```python
from build123d import *

# Parameters (mm, degrees)
SKETCH1_R               = 16
SKETCH1_R_2             = 2
BOSS_EXTRUDE1_DEPTH     = 5
SKETCH2_R               = 7.5
BOSS_EXTRUDE2_DEPTH     = 18.5
CUT_EXTRUDE1_DEPTH      = 33.622844756
CUT_EXTRUDE1_DEPTH_BACK = 33.622844756
SKETCH3_R               = 4


with BuildPart() as part:
    # Sketch1 → Boss-Extrude1 (new body)
    with BuildSketch(Plane(origin=(0, 0, 0), x_dir=(0, 0, -1), z_dir=(1, 0, 0))):
        Circle(SKETCH1_R)
        with Locations((0, 12)):
            Circle(SKETCH1_R_2, mode=Mode.SUBTRACT)
        with Locations((12, 0)):
            Circle(SKETCH1_R_2, mode=Mode.SUBTRACT)
        with Locations((0, -12)):
            Circle(SKETCH1_R_2, mode=Mode.SUBTRACT)
        with Locations((-12, 0)):
            Circle(SKETCH1_R_2, mode=Mode.SUBTRACT)
    extrude(amount=BOSS_EXTRUDE1_DEPTH)

    # Sketch2 → Boss-Extrude2 (add)
    with BuildSketch(Plane(origin=(5, 0, 0), x_dir=(0, 0, -1), z_dir=(1, 0, 0))):
        Circle(SKETCH2_R)
    extrude(amount=BOSS_EXTRUDE2_DEPTH)

    # Sketch3 → Cut-Extrude1 (cut, two sides: drawn at the far end of the back side and taken through both)
    with BuildSketch(Plane.ZY.offset(-CUT_EXTRUDE1_DEPTH_BACK)):
        Circle(SKETCH3_R)
    extrude(amount=CUT_EXTRUDE1_DEPTH + CUT_EXTRUDE1_DEPTH_BACK, mode=Mode.SUBTRACT)


solid = part.part
```
Input: part model. Units: mm. Frame: model coordinates. A direction names the side the tool comes from. Round coordinates to 2 decimals unless told otherwise and drop trailing zeros. Write each loop counter-clockwise with the first axis right and the second up, starting at its lowest first coordinate (ties: lowest second). Pieces come first, ordered by that corner, then holes. Notation, with made-up numbers: M 14,12 L 42,12 A13 ccw 42,24 Z; hole C 65.25,82.25 d9. An arc over 180 degrees is marked long. Write each question's results on one line, items separated by ' | '.
Q1. Draft query along Y for faces 3 (the face through (2.46, -15.62, 3.47)), 4 (the face through (23.5, -3, -3)), 5 (the face through (11.914, -3.905, -0.867)). Return one class per face: released by +Y, released by -Y, zero draft, split by the parting line, or undercut.
Results:
face 3: split by the parting line | face 4: zero draft | face 5: undercut
Q2. Access query for faces 1 (the face through (14.12, 0.33, 7.493)), 2 (the face through (2, 14, 0)). Directions: +Z, -Z, +X, -X, +Y, -Y. A direction counts if a zero-diameter tool reaches every point of the face in a straight line with its end or side. Return the directions, or none.
Results:
face 1: +X | face 2: +X, -X
Q3. Section query C-C (z = 12). Return loops of the section in (x, y).
Results:
outline: M 0,-10.58 L 5,-10.58 L 5,-2 L 0,-2 Z; M 0,2 L 5,2 L 5,10.58 L 0,10.58 Z
Q4. Pin query (flat end, axial travel): P1, Ø2, axis at x = 18, z = 3.5, coming from the +Y side; P2, Ø12, axis at x = 20, y = -10.5, coming from the -Z side; P3, Ø4, axis at x = 10.5, y = 2.5, coming from the -Z side. Return the tip coordinate at first contact, or that it passes through.
Results:
P1: stops at y = 7.07 | P2: stops at z = -6 | P3: stops at z = -7.48
Q5. Section query A-A (z = 0). Return loops of the section in (x, y), and give its area (4 significant figures).
Results:
outline: M 0,-16 L 5,-16 L 5,-14 L 0,-14 Z; M 0,-10 L 5,-10 L 5,-7.5 L 23.5,-7.5 L 23.5,-4 L 0,-4 Z; M 0,4 L 23.5,4 L 23.5,7.5 L 5,7.5 L 5,10 L 0,10 Z; M 0,14 L 5,14 L 5,16 L 0,16 Z | area: 209.5 mm^2
Q6. Line query: line 1 along Y through (x, z) = (1.5, 0); line 2 along X through (y, z) = (-11, -10); line 3 along Y through (x, z) = (17.75, 0). Output: solid intervals per line, ascending.
Results:
line 1: y = -16 to -14, -10 to -4, 4 to 10, 14 to 16 | line 2: x = 0 to 5 | line 3: y = -7.5 to -4, 4 to 7.5
Q7. Section query D-D (x = 2.25). Return loops of the section in (y, z).
Results:
outline: C 0,0 d32; hole C -12,0 d4; hole C 0,0 d8; hole C 0,-12 d4; hole C 0,12 d4; hole C 12,0 d4
